from build123d import *

# Parameters (mm, degrees)
BOSS_EXTRUDE1_DEPTH = 545
CUT_EXTRUDE2_DEPTH  = 10
CUT_EXTRUDE3_DEPTH  = 10


with BuildPart() as part:
    # Sketch1 → Boss-Extrude1 (new body)
    with BuildSketch(Plane.XY):
        Polygon((-9.451520251, 23.80952381), (-9.451520251, -26.19047619), (15.548479749, -26.19047619), (15.548479749, -23.69047619), (-6.951520251, -23.69047619), (-6.951520251, 23.80952381), align=None)
    extrude(amount=BOSS_EXTRUDE1_DEPTH)

    # Sketch3 → Cut-Extrude2 (cut)
    with BuildSketch(Plane(origin=(0, -23.69047619, 0), x_dir=(1, 0, 0), z_dir=(0, 1, 0))):
        with BuildLine():
            Line((0.57076558, -242.790014276), (0.57076558, -223.790014276))
            ThreePointArc((0.57076558, -223.790014276), (4.07076558, -220.926188945), (7.57076558, -223.790014276))
            Line((7.57076558, -223.790014276), (7.57076558, -242.790014276))
            ThreePointArc((7.57076558, -242.790014276), (4.07076558, -246.37195288), (0.57076558, -242.790014276))
        make_face()
        with BuildLine():
            Line((0.807679204, -169.35276274), (0.808591774, -150.352762761))
            ThreePointArc((0.808591774, -150.352762761), (4.309142051, -146.853313591), (7.808591221, -150.353863868))
            Line((7.808591221, -150.353863868), (7.809609956, -169.355340241))
            ThreePointArc((7.809609956, -169.355340241), (4.307302192, -173.000725763), (0.807679204, -169.35276274))
        make_face()
        with BuildLine():
            Line((0.583868221, -24), (0.583868221, -6))
            ThreePointArc((0.583868221, -6), (4.083868221, -2.5), (7.583868221, -6))
            Line((7.583868221, -6), (7.583868221, -24))
            ThreePointArc((7.583868221, -24), (4.083868221, -27.222249808), (0.583868221, -24))
        make_face()
        with BuildLine():
            Line((0.55068367, -316.822260412), (0.55068367, -297.822260412))
            ThreePointArc((0.55068367, -297.822260412), (4.05068367, -294.370676122), (7.55068367, -297.822260412))
            Line((7.55068367, -297.822260412), (7.55068367, -316.822260412))
            ThreePointArc((7.55068367, -316.822260412), (4.05068367, -320.404199017), (0.55068367, -316.822260412))
        make_face()
        with BuildLine():
            Line((0.548436659, -390.854506502), (0.548436659, -371.854506502))
            ThreePointArc((0.548436659, -371.854506502), (4.048436659, -368.402922212), (7.548436659, -371.854506502))
            Line((7.548436659, -371.854506502), (7.548436659, -390.854506502))
            ThreePointArc((7.548436659, -390.854506502), (4.048436659, -394.436445107), (0.548436659, -390.854506502))
        make_face()
        with BuildLine():
            Line((0.543910271, -464.886752452), (0.543910271, -445.886752452))
            ThreePointArc((0.543910271, -445.886752452), (4.043910271, -442.435168162), (7.543910271, -445.886752452))
            Line((7.543910271, -445.886752452), (7.543910271, -464.886752452))
            ThreePointArc((7.543910271, -464.886752452), (4.043910271, -468.468691057), (0.543910271, -464.886752452))
        make_face()
        with BuildLine():
            Line((0.482021973, -538.918998588), (0.482021973, -519.918998588))
            ThreePointArc((0.482021973, -519.918998588), (3.982021973, -516.467414298), (7.482021973, -519.918998588))
            Line((7.482021973, -519.918998588), (7.482021973, -538.918998588))
            ThreePointArc((7.482021973, -538.918998588), (3.982021973, -542.500937193), (0.482021973, -538.918998588))
        make_face()
        with BuildLine():
            Line((0.799787986, -95.209226687), (0.798633115, -76.892344291))
            ThreePointArc((0.798633115, -76.892344291), (4.297807626, -73.191635658), (7.798672507, -76.890745244))
            Line((7.798672507, -76.890745244), (7.801718738, -95.211804188))
            ThreePointArc((7.801718738, -95.211804188), (4.299410974, -98.857189711), (0.799787986, -95.209226687))
        make_face()
    extrude(amount=-CUT_EXTRUDE2_DEPTH, mode=Mode.SUBTRACT)

    # Sketch2 → Cut-Extrude3 (cut)
    with BuildSketch(Plane(origin=(-6.951520251, 0, 0), x_dir=(0, 0, -1), z_dir=(1, 0, 0))):
        with BuildLine():
            Line((-523.677073705, 11.34825395), (-464.779022926, 11.34825395))
            ThreePointArc((-464.779022926, 11.34825395), (-453.273357193, -0.157411783), (-464.779022926, -11.663077517))
            Line((-464.779022926, -11.663077517), (-523.677073705, -11.663077517))
            ThreePointArc((-523.677073705, -11.663077517), (-535.182739439, -0.157411783), (-523.677073705, 11.34825395))
        make_face()
        with BuildLine():
            Line((-364.779022926, 11.087774361), (-305.880972148, 11.087774361))
            ThreePointArc((-305.880972148, 11.087774361), (-294.548021848, -0.417891372), (-305.880972148, -11.923557106))
            Line((-305.880972148, -11.923557106), (-364.779022926, -11.923557106))
            ThreePointArc((-364.779022926, -11.923557106), (-376.28468866, -0.417891372), (-364.779022926, 11.087774361))
        make_face()
        with BuildLine():
            Line((-241.055003683, 11.260273997), (-182.156952904, 11.260273997))
            ThreePointArc((-182.156952904, 11.260273997), (-170.65128717, -0.245391736), (-182.156952904, -11.75105747))
            Line((-182.156952904, -11.75105747), (-241.055003683, -11.75105747))
            ThreePointArc((-241.055003683, -11.75105747), (-252.560669416, -0.245391736), (-241.055003683, 11.260273997))
        make_face()
        with BuildLine():
            Line((-82.156952904, 11.402162448), (-23.258902125, 11.402162448))
            ThreePointArc((-23.258902125, 11.402162448), (-11.753236392, -0.103503285), (-23.258902125, -11.609169019))
            Line((-23.258902125, -11.609169019), (-82.156952904, -11.609169019))
            ThreePointArc((-82.156952904, -11.609169019), (-93.662618637, -0.103503285), (-82.156952904, 11.402162448))
        make_face()
    extrude(amount=-CUT_EXTRUDE3_DEPTH, mode=Mode.SUBTRACT)


solid = part.part
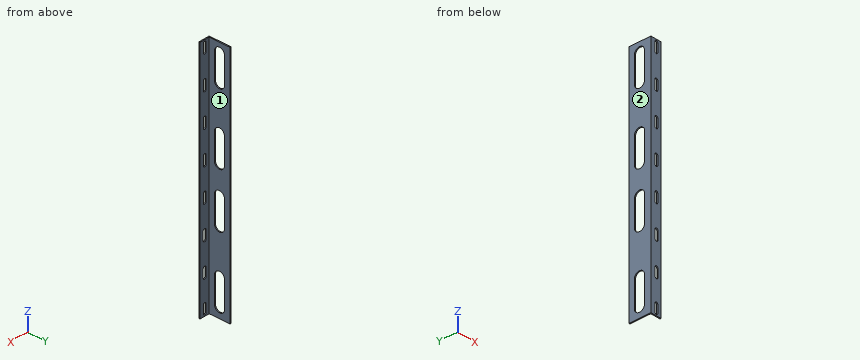
Geometry: final body of the model. Coordinates: model frame, mm. Face numbers are marked on the shaded views. A direction names the side the tool comes from. Round coordinates to 2 decimals unless told otherwise and drop trailing zeros. Write each loop counter-clockwise with the first axis right and the second up, starting at its lowest first coordinate (ties: lowest second). Pieces come first, ordered by that corner, then holes. Notation, with made-up numbers: M 55,42 L 76,42 A22 cw 76,57 Z; hole C 64.25,4 d8. An arc over 180 degrees is marked long. Write item = value, one per line.
Item 1: Access query for the marked faces 1 and 2. Directions: +Z, -Z, +X, -X, +Y, -Y. A direction counts if a zero-diameter tool reaches every point of the face in a straight line with its end or side. Return the directions, or none.
Findings:
face_1 = +Z, -Z, +X, +Y
face_2 = +Z, -Z, -X, +Y, -Y
Item 2: Section query A-A on y = -4. Return loops of the section in (x, z).
Findings:
outline = M -9.45,0 L -6.95,0 L -6.95,12.43 L -9.45,12.43 Z; M -9.45,92.98 L -6.95,92.98 L -6.95,171.28 L -9.45,171.28 Z; M -9.45,251.93 L -6.95,251.93 L -6.95,295.12 L -9.45,295.12 Z; M -9.45,375.71 L -6.95,375.71 L -6.95,453.93 L -9.45,453.93 Z; M -9.45,534.52 L -6.95,534.52 L -6.95,545 L -9.45,545 Z
Item 3: Section query B-B on z = 119.5. Return loops of the section in (x, y), then the cut area to 3 significant figures.
Findings:
outline = M -9.45,-26.19 L 15.55,-26.19 L 15.55,-23.69 L -6.95,-23.69 L -6.95,23.81 L -9.45,23.81 Z
area = 181 mm^2
Item 4: Pin query (flat end, axial travel): P1, Ø8, axis at y = -6, z = 88.5, coming from the -X side; P2, Ø3, axis at x = 10, z = 260, coming from the +Y side. Return the tip coordinate at first contact, or that it passes through.
Findings:
P1 = -9.45
P2 = -23.69
Item 5: Material intervals for line 1 along X through (y, z) = (-23, 298); line 2 along Y through (x, z) = (-7.5, 479.5); line 3 along Y through (x, z) = (12.5, 435), sorted ascending. Write a range as [from, to].
Findings:
line_1 = [-9.45, -6.95]
line_2 = [-26.19, -11.66], [11.35, 23.81]
line_3 = [-26.19, -23.69]
